The model under review builds one solid part; all positions refer to its coordinate system, in mm. Coordinates: 2 decimals unless noted, no trailing zeros. Loops run counter-clockwise (first coordinate to the right, second up) from the corner with the lowest first, then second, coordinate; pieces in that order, holes last. Notation, with made-up numbers: M 11.25,13.5 L 37.25,13.5 A14 ccw 37.25,28.5 Z; hole C 14.5,73.25 d8. An arc over 180 degrees is marked long. Write item = value, one per line. Start each with the question number.
Q1. We need section A-A on x = -3. Give the boundary of the cut face in (y, z), and give its area (3 significant figures).
Q2. We need section B-B on z = -15. Give the boundary of the cut face in (x, y), and give its area (3 significant figures).
Q3. Clearance check with flat-ended pins moving along their axes: pin 1 Ø4.5 at (x, z) = (-6.2, -49.5) entering from +Y; pin 2 Ø1 at (x, y) = (-6, 30) entering from -Z; pin 3 Ø1.6 at (x, y) = (-5.5, 30.5) entering from +Z; pin 4 Ø2.5 at (x, z) = (-6.2, 49.5) entering from -Y. State where each tip first meets the part, or that it passes through.
Q4. Wall thickness on probe 1 along X at (y, z) = (30.9, -49.5); probe 2 along Z at (x, y) = (-9, 30.5); probe 3 along X at (y, z) = (31.5, 25.5): over which ranges is each line inside the solid? List them lowest first.
Q5. We need section C-C on y = 36.75. Give the boundary of the cut face in (x, z), and give its area (3 significant figures).
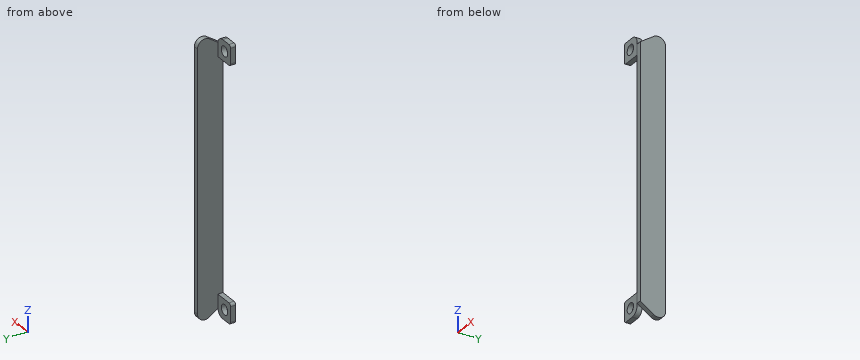
from build123d import *

# Parameters (mm, degrees)
BASE_FLANGE1_DEPTH               = 2
FILLET1_R                        = 3
BOSS_EXTRUDE1_START              = 29.3979
BOSS_EXTRUDE1_DEPTH              = 2
F_4_0_START                      = 29.397900258
F_4_0_4_DIAMETER_HOLE1_OUTLINE_R = 2
F_4_0_4_DIAMETER_HOLE1_DEPTH     = 2
FILLET2_R                        = 3


# Read off the part's stored shape, not the designer's step: Ø4.0 (4) Diameter Hole1
# Sheet-metal steps are written as plain solids
with BuildPart() as part:
    # Sketch1 → Base-Flange1 (new body)
    with BuildSketch(Plane(origin=(0, 0, 0), x_dir=(0, 0, -1), z_dir=(1, 0, 0))):
        Polygon((49.662255386, 29.397900258), (56.5, 39.397900258), (-56.5, 39.397900258), (-49.662255386, 29.397900258), align=None)
    extrude(amount=-BASE_FLANGE1_DEPTH)

    # Fillet1
    fillet1_edges = [part.edges().sort_by_distance(p)[0] for p in [
        (-1, 39.397900258, 56.5),
        (-1, 39.397900258, -56.5),
    ]]
    fillet(fillet1_edges, radius=FILLET1_R)

    # Sketch2 → Boss-Extrude1 (add)
    with BuildSketch(Plane(origin=(0, 0, 0), x_dir=(1, 0, 0), z_dir=(0, 1, 0)).offset(BOSS_EXTRUDE1_START)):
        with BuildLine():
            Line((-2, 53.5), (-9, 53.5))
            ThreePointArc((-9, 53.5), (-9.707106781, 53.207106781), (-10, 52.5))
            Line((-10, 52.5), (-10, 46.5))
            ThreePointArc((-10, 46.5), (-9.707106781, 45.792893219), (-9, 45.5))
            Line((-9, 45.5), (-2, 45.5))
            Line((-2, 45.5), (-2, 53.5))
        make_face()
        with BuildLine():
            Line((-10, -52.5), (-10, -46.5))
            ThreePointArc((-10, -46.5), (-9.707106781, -45.792893219), (-9, -45.5))
            Line((-9, -45.5), (-2, -45.5))
            Line((-2, -45.5), (-2, -53.5))
            Line((-2, -53.5), (-9, -53.5))
            ThreePointArc((-9, -53.5), (-9.707106781, -53.207106781), (-10, -52.5))
        make_face()
    extrude(amount=BOSS_EXTRUDE1_DEPTH)

    # Ø4.0 (4) Diameter Hole1 outline → Ø4.0 (4) Diameter Hole1 (cut)
    with BuildSketch(Plane(origin=(0, 0, 0), x_dir=(1, 0, 0), z_dir=(0, 1, 0)).offset(F_4_0_START)):
        with Locations((-6.20230671, -49.5)):
            Circle(F_4_0_4_DIAMETER_HOLE1_OUTLINE_R)
        with Locations((-6.20230671, 49.5)):
            Circle(F_4_0_4_DIAMETER_HOLE1_OUTLINE_R)
    extrude(amount=F_4_0_4_DIAMETER_HOLE1_DEPTH, mode=Mode.SUBTRACT)

    # Fillet2
    # the kernel refuses this fillet: 3 mm, written as the material it takes off along each edge
    with BuildSketch(Plane(origin=(-2, 21.8979, -53.5), x_dir=(0, 0, 1), z_dir=(0, 1, 0))) as fillet2_piece_1:
        with BuildLine():
            CenterArc((FILLET2_R, -FILLET2_R), FILLET2_R, 90, 90)
            Line((0, -FILLET2_R), (0, 0))
            Line((0, 0), (FILLET2_R, 0))
        make_face()
    extrude(amount=17, mode=Mode.SUBTRACT)
    with BuildSketch(Plane(origin=(-2, 21.8979, 53.5), x_dir=(0, 0, -1), z_dir=(0, 1, 0))) as fillet2_piece_2:
        with BuildLine():
            CenterArc((FILLET2_R, FILLET2_R), FILLET2_R, 180, 90)
            Line((0, FILLET2_R), (0, 0))
            Line((0, 0), (FILLET2_R, 0))
        make_face()
    extrude(amount=17, mode=Mode.SUBTRACT)


solid = part.part
Returned:
q1.outline = M 29.4,-52.74 L 31.4,-52.74 L 31.4,-45.5 L 29.4,-45.5 Z; M 29.4,45.5 L 31.4,45.5 L 31.4,52.74 L 29.4,52.74 Z
q1.area = 28.9 mm^2
q2.outline = M -2,29.4 L 0,29.4 L 0,39.4 L -2,39.4 Z
q2.area = 20.0 mm^2
q3.pin_1 = 31.4
q3.pin_2 = -53.5
q3.pin_3 = 53.5
q3.pin_4 = through
q4.probe_1 = -10 to -8.2, -4.2 to 0
q4.probe_2 = -53.5 to -45.5, 45.5 to 53.5
q4.probe_3 = -2 to 0
q5.outline = M -2,-53.79 L 0,-53.79 L 0,53.79 L -2,53.79 Z
q5.area = 215 mm^2
